```python
from build123d import *

# Parameters (mm, degrees)
SKETCH1_W            = 308.08168
SKETCH1_H            = 3.175
BOSS_EXTRUDE1_DEPTH  = 267.83
SKETCH3_W            = 267.83
SKETCH3_H            = 3.175
BOSS_EXTRUDE3_DEPTH  = 3.175
SKETCH4_W            = 50.8889
SKETCH4_H            = 3.175
BOSS_EXTRUDE4_DEPTH  = 267.83
CUT_EXTRUDE1_DEPTH   = 340.191055801
SKETCH17_W           = 267.83
SKETCH17_H           = 3.175
BOSS_EXTRUDE5_DEPTH  = 3.175
CUT_EXTRUDE3_DEPTH   = 340.191055801
SKETCH25_R           = 3.175
CUT_EXTRUDE8_DEPTH   = 3.175
SKETCH27_R           = 5
CUT_EXTRUDE9_DEPTH   = 340.191055801
SKETCH30_W           = 80
SKETCH30_H           = 3.175
BOSS_EXTRUDE6_DEPTH  = 3.175
SKETCH31_R           = 1.5875
CUT_EXTRUDE10_DEPTH  = 340.191055801
LPATTERN1_COUNT      = 3
LPATTERN1_PITCH      = 58
M4_CLEARANCE_HOLE1_D = 4.8


with BuildPart() as part:
    # Sketch1 → Boss-Extrude1 (new body)
    with BuildSketch(Plane.XY):
        Rectangle(SKETCH1_W, SKETCH1_H)
    extrude(amount=BOSS_EXTRUDE1_DEPTH)

    # Sketch3 → Boss-Extrude3 (add)
    with BuildSketch(Plane(origin=(154.04084, 0, 0), x_dir=(0, 0, -1), z_dir=(1, 0, 0))):
        with Locations((-133.915, 0)):
            Rectangle(SKETCH3_W, SKETCH3_H)
    extrude(amount=BOSS_EXTRUDE3_DEPTH)

    # Sketch4 → Boss-Extrude4 (add)
    with BuildSketch(Plane.XY.offset(267.83)):
        with Locations((182.66029, 0)):
            Rectangle(SKETCH4_W, SKETCH4_H)
    extrude(amount=-BOSS_EXTRUDE4_DEPTH)

    # Sketch6 → Cut-Extrude1 (cut, through all)
    with BuildSketch(Plane(origin=(0, 1.5875, 0), x_dir=(1, 0, 0), z_dir=(0, 1, 0))):
        Polygon((208.10474, -240.606362049), (106.50474, -267.83), (208.10474, -267.83), align=None)
    extrude(amount=-CUT_EXTRUDE1_DEPTH, mode=Mode.SUBTRACT)

    # Sketch17 → Boss-Extrude5 (add)
    with BuildSketch(Plane.ZY.offset(154.04084)):
        with Locations((133.915, 0)):
            Rectangle(SKETCH17_W, SKETCH17_H)
    extrude(amount=BOSS_EXTRUDE5_DEPTH)

    # Sketch11 → Cut-Extrude3 (cut, through all)
    with BuildSketch(Plane.XZ.offset(1.5875)):
        Polygon((-157.21584, 241.2743), (-84.254653892, 267.83), (-157.21584, 267.83), align=None)
    extrude(amount=-CUT_EXTRUDE3_DEPTH, mode=Mode.SUBTRACT)

    # Sketch25 → Cut-Extrude8 (cut)
    with BuildSketch(Plane.XZ.offset(1.5875)):
        with Locations(Location((-115.322188641, 247.921359373, 0), (0, 0, 270))):
            Circle(SKETCH25_R)
        with Locations(Location((-50.97526, 258.94, 0), (0, 0, 270))):
            Circle(SKETCH25_R)
        with Locations(Location((11.25474, 258.94, 0), (0, 0, 270))):
            Circle(SKETCH25_R)
        with Locations(Location((73.48474, 258.94, 0), (0, 0, 270))):
            Circle(SKETCH25_R)
        with Locations(Location((172.54474, 242.09298883, 0), (0, 0, 270))):
            Circle(SKETCH25_R)
        with Locations(Location((131.90474, 252.982444011, 0), (0, 0, 270))):
            Circle(SKETCH25_R)
    extrude(amount=-CUT_EXTRUDE8_DEPTH, mode=Mode.SUBTRACT)

    # Sketch27 → Cut-Extrude9 (cut, through all)
    with BuildSketch(Plane.XZ.offset(1.5875)):
        with Locations(Location((172.48674, 137.774823778, 0), (0, 0, 270))):
            Circle(SKETCH27_R)
        with Locations(Location((183.48674, 137.774823778, 0), (0, 0, 270))):
            Circle(SKETCH27_R)
        with Locations(Location((194.48674, 137.774823778, 0), (0, 0, 270))):
            Circle(SKETCH27_R)
        with Locations(Location((194.48674, 126.774823778, 0), (0, 0, 270))):
            Circle(SKETCH27_R)
        with Locations(Location((194.48674, 115.774823778, 0), (0, 0, 270))):
            Circle(SKETCH27_R)
        with Locations(Location((183.48674, 126.774823778, 0), (0, 0, 270))):
            Circle(SKETCH27_R)
        with Locations(Location((183.48674, 115.774823778, 0), (0, 0, 270))):
            Circle(SKETCH27_R)
        with Locations(Location((172.48674, 115.774823778, 0), (0, 0, 270))):
            Circle(SKETCH27_R)
        with Locations(Location((172.48674, 126.774823778, 0), (0, 0, 270))):
            Circle(SKETCH27_R)
        with Locations(Location((194.48674, 71.774823778, 0), (0, 0, 270))):
            Circle(SKETCH27_R)
        with Locations(Location((194.48674, 60.774823778, 0), (0, 0, 270))):
            Circle(SKETCH27_R)
        with Locations(Location((194.48674, 49.774823778, 0), (0, 0, 270))):
            Circle(SKETCH27_R)
        with Locations(Location((183.48674, 71.774823778, 0), (0, 0, 270))):
            Circle(SKETCH27_R)
        with Locations(Location((183.48674, 60.774823778, 0), (0, 0, 270))):
            Circle(SKETCH27_R)
        with Locations(Location((183.48674, 49.774823778, 0), (0, 0, 270))):
            Circle(SKETCH27_R)
        with Locations(Location((172.48674, 49.774823778, 0), (0, 0, 270))):
            Circle(SKETCH27_R)
        with Locations(Location((172.48674, 60.774823778, 0), (0, 0, 270))):
            Circle(SKETCH27_R)
        with Locations(Location((172.48674, 71.774823778, 0), (0, 0, 270))):
            Circle(SKETCH27_R)
    extrude(amount=-CUT_EXTRUDE9_DEPTH, mode=Mode.SUBTRACT)

    # Sketch30 → Boss-Extrude6 (add)
    with BuildSketch(Plane(origin=(0, 0, 0), x_dir=(-1, 0, 0), z_dir=(0, 0, -1))):
        with Locations((-2.78399998, 0)):
            Rectangle(SKETCH30_W, SKETCH30_H)
    extrude(amount=BOSS_EXTRUDE6_DEPTH)

    # Sketch31 → Cut-Extrude10 (cut, symmetric)
    with BuildSketch(Plane.XZ.offset(1.5875)):
        with Locations(Location((183.48674, 151.774823778, 0), (0, 0, 270))):
            Circle(SKETCH31_R)
    cut_extrude10 = extrude(amount=CUT_EXTRUDE10_DEPTH, both=True, mode=Mode.SUBTRACT)

    # LPattern1: Cut-Extrude10 ×3
    with Locations(*[(0, 0, -i * LPATTERN1_PITCH) for i in range(1, LPATTERN1_COUNT)]):
        add(cut_extrude10, mode=Mode.SUBTRACT)

    # M4 Clearance Hole1 (through all)
    with Locations(Plane.XZ.offset(1.5875)):
        with Locations((180.96500002, 176.776), (-97.77095, 213.2849914), (3.82905, 213.2849914), (105.42905, 213.2849914)):
            Hole(M4_CLEARANCE_HOLE1_D / 2)


solid = part.part
```
Geometry check sheet. Reference: the model listing, model coordinates, mm. Give positions to 0.01 mm unless a question says otherwise; leave off trailing zeros. Order: outer loops, then holes, each group sorted by start corner. A loop starts at its lowest first (then second) coordinate and runs counter-clockwise, first axis right, second up.
1. Thickness scan on L1, parallel to X at y = 0.8, z = 49.5; L2, parallel to X at y = -0.2, z = 50.5; L3, parallel to Z at x = -46, y = -1.35. Record the ranges inside material, lowest first.
2. Section check B-B, the plane y = 0.4. Give the number of separate pieces and of enclosed holes in the cut face, and give its area (3 significant figures).
3. Section check A-A, the plane z = 127. Enter the section's corners in (x, y).
4. Release check for a two-part mould opening along Z. For faces 1 (the face through (195.989, -0.022, 133.006)), 2 (the face through (28, 1.588, 130)), 3 (the face through (-121.246, -0.022, 254.366)), 4 (the face through (182, 0, 56)) record: pulls with the +Z half, pulls with the -Z half, needs draft (parallel to the pull), parting line crosses it, or undercut.
Values follow:
1. L1: x = -157.22 to 167.49, 177.48 to 178.49, 188.48 to 189.49, 199.48 to 208.1
1. L2: x = -157.22 to 167.54, 177.43 to 178.54, 188.43 to 189.54, 199.43 to 208.1
1. L3: z = 0 to 267.83
2. separate pieces: 1
2. enclosed holes: 31
2. area: 94,000 mm2
3. outline: (-157.22, -1.59) - (167.49, -1.59) - (167.49, 1.59) - (-157.22, 1.59) - close; (177.48, -1.59) - (178.49, -1.59) - (178.49, 1.59) - (177.48, 1.59) - close; (188.48, -1.59) - (189.49, -1.59) - (189.49, 1.59) - (188.48, 1.59) - close; (199.48, -1.59) - (208.1, -1.59) - (208.1, 1.59) - (199.48, 1.59) - close
4. face 1: undercut
4. face 2: needs draft
4. face 3: pulls with the +Z half
4. face 4: undercut
